```python
from build123d import *

# Parameters (mm, degrees)
F0_W           = 76.2
F0_H           = 12.7
F1_DEPTH       = 12.7
F2_D           = 6.5278
F3_D           = 6.5278
F5_D           = 4.4
F5_CBORE_D     = 8.25
F5_CBORE_DEPTH = 4
F6_D           = 4.4
F6_CBORE_D     = 8.25
F6_CBORE_DEPTH = 4


with BuildPart() as f1:
    # F0 (on Top) → F1 (new body)
    with BuildSketch(Plane.XY):
        Rectangle(F0_W, F0_H)
    extrude(amount=F1_DEPTH)

    # F2 (through all)
    with Locations(Plane(origin=(0, 0, 0), x_dir=(1, 0, 0), z_dir=(0, 0, -1))):
        with Locations((-19.05, 0)):
            Hole(F2_D / 2)

    # F3 (through all)
    with Locations(Plane(origin=(0, 0, 0), x_dir=(1, 0, 0), z_dir=(0, 0, -1))):
        with Locations((19.05, 0)):
            Hole(F3_D / 2)

    # F5 (through all)
    with Locations(Plane.XZ.offset(6.35)):
        with Locations((-6.985, 5.08)):
            CounterBoreHole(F5_D / 2, F5_CBORE_D / 2, F5_CBORE_DEPTH)

    # F6 (through all)
    with Locations(Plane.XZ.offset(6.35)):
        with Locations((6.985, 5.08)):
            CounterBoreHole(F6_D / 2, F6_CBORE_D / 2, F6_CBORE_DEPTH)


solid = f1.part
```
Read the model definition and answer for the solid it produces. Units are mm, in the model's axes. A direction names the side the tool comes from. Coordinates: 2 decimals unless noted, no trailing zeros. Loops run counter-clockwise (first coordinate to the right, second up) from the corner with the lowest first, then second, coordinate; pieces in that order, holes last. Notation, with made-up numbers: (34, -30) -> (91, -30) arc R29 ccw to (91, 3) -> close; hole circle Ø9 at (22.5, -5). An arc over 180 degrees is marked (long way). Return JSON: item names as keys, results as strings.
Item 1: Find section C-C (y = -4). Determine the outline of the cut face in (x, z) (3 decimals), plus the area to 3 significant figures.
Answers:
{"outline": "(-38.1, 0) -> (38.1, 0) -> (38.1, 12.7) -> (-38.1, 12.7) -> close; hole circle Ø8.25 at (-6.985, 5.08); hole circle Ø8.25 at (6.985, 5.08)", "area": "861 mm2"}
Item 2: For a pull along Z with two mould halves and no side action, classify faces 1 (the flat face through (-1, 0, 0)), 2 (the cylindrical face through (10.795, -4.378, 3.5)), 3 (the cylindrical face through (22.31, -0.14, 6.44)) as +Z half, -Z half, draft (parallel to the pull), parting line (faces both ways), or undercut.
Answers:
{"face 1": "-Z half", "face 2": "undercut", "face 3": "draft"}
Item 3: Find the intervals of material crossed by probe 1 along X at (y, z) = (-0.25, 8.25); probe 2 along X at (y, z) = (-0.5, 3.5); probe 3 along X at (y, z) = (-5, 3.75), in increasing order.
Answers:
{"probe 1": "x = -38.1 to -22.3, -15.8 to 15.8, 22.3 to 38.1", "probe 2": "x = -38.1 to -22.28, -15.82 to -8.52, -5.45 to 5.45, 8.52 to 15.82, 22.28 to 38.1", "probe 3": "x = -38.1 to -10.89, -3.08 to 3.08, 10.89 to 38.1"}
Item 4: Find section B-B (x = -19.05). Determine the outline of the cut face in (y, z), plus the area to 3 significant figures.
Answers:
{"outline": "(-6.35, 0) -> (-3.26, 0) -> (-3.26, 12.7) -> (-6.35, 12.7) -> close; (3.26, 0) -> (6.35, 0) -> (6.35, 12.7) -> (3.26, 12.7) -> close", "area": "78.4 mm2"}
Item 5: Find section D-D (x = 21). Determine the outline of the cut face in (y, z), plus the area to 3 significant figures.
Answers:
{"outline": "(-6.35, 0) -> (-2.62, 0) -> (-2.62, 12.7) -> (-6.35, 12.7) -> close; (2.62, 0) -> (6.35, 0) -> (6.35, 12.7) -> (2.62, 12.7) -> close", "area": "94.8 mm2"}
Item 6: Flat-ended cylindrical pins translate along their axes: P1, Ø2.5, axis at x = 5.5, z = 6.5, coming from the -Y side; P2, Ø3.5, axis at x = -6.985, z = 5.08, coming from the -Y side; P3, Ø5, axis at x = 23.5, y = -1.5, coming from the -Z side. Find the tip coordinate at first contact, or state that the pin passes through.
Answers:
{"P1": "stops at y = -2.35", "P2": "passes through", "P3": "stops at z = 0"}
Item 7: Find section A-A (z = 5.08). Determine the outline of the cut face in (x, y) (3 decimals).
Answers:
{"outline": "(-38.1, -6.35) -> (-11.11, -6.35) -> (-11.11, -2.35) -> (-9.185, -2.35) -> (-9.185, 6.35) -> (-38.1, 6.35) -> close; (-4.785, -2.35) -> (-2.86, -2.35) -> (-2.86, -6.35) -> (2.86, -6.35) -> (2.86, -2.35) -> (4.785, -2.35) -> (4.785, 6.35) -> (-4.785, 6.35) -> close; (9.185, -2.35) -> (11.11, -2.35) -> (11.11, -6.35) -> (38.1, -6.35) -> (38.1, 6.35) -> (9.185, 6.35) -> close; hole circle Ø6.528 at (-19.05, 0); hole circle Ø6.528 at (19.05, 0)"}
Item 8: For faces 4 (the flat face through (38.1, 0, 6)), 5 (the flat face through (9, -2.35, 3)), determine the directions among +Z, -Z, +X, -X, +Y, -Y from which every point of the face is accessible in a straight line to the end or side of a thin tool.
Answers:
{"face 4": "+Z, -Z, +X, +Y, -Y", "face 5": "-Y"}
